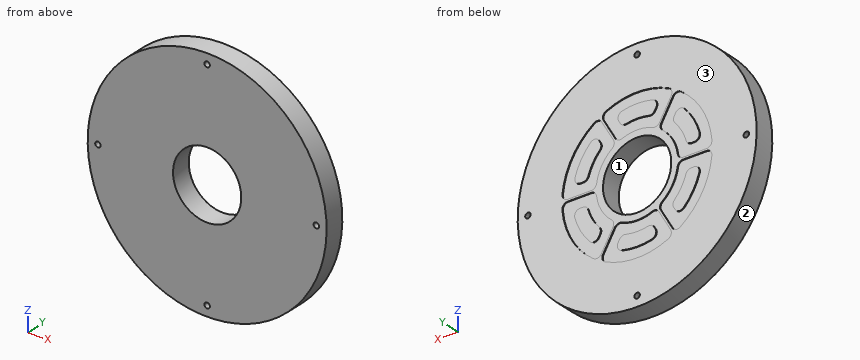
from build123d import *

# Parameters (mm, degrees)
SKETCH2_R           = 175
BOSS_EXTRUDE1_DEPTH = 15
SKETCH3_R           = 4
SKETCH3_R_2         = 50
CUT_EXTRUDE1_DEPTH  = 30
CUT_EXTRUDE3_DEPTH  = 1
CIRPATTERN2_COUNT   = 6


with BuildPart() as part:
    # Sketch2 → Boss-Extrude1 (new, symmetric)
    with BuildSketch(Plane(origin=(0, 0, 0), x_dir=(1, 0, 0), z_dir=(0, 1, 0))):
        with Locations(Location((0, 0, 0), (0, 0, 270))):
            Circle(SKETCH2_R)
    extrude(amount=BOSS_EXTRUDE1_DEPTH, both=True)

    # Sketch3 → Cut-Extrude1 (cut)
    with BuildSketch(Plane(origin=(0, 15, 0), x_dir=(1, 0, 0), z_dir=(0, 1, 0))):
        with Locations(Location((0, 160, 0), (0, 0, 270))):
            Circle(SKETCH3_R)
        with Locations(Location((0, -160, 0), (0, 0, 90))):
            Circle(SKETCH3_R)
        with Locations(Location((-160, 0, 0), (0, 0, 270))):
            Circle(SKETCH3_R)
        with Locations(Location((160, 0, 0), (0, 0, 90))):
            Circle(SKETCH3_R)
        with Locations(Location((0, 0, 0), (0, 0, 270))):
            Circle(SKETCH3_R_2)
    extrude(amount=-CUT_EXTRUDE1_DEPTH, mode=Mode.SUBTRACT)

    # Sketch4 → Cut-Extrude3 (cut)
    with BuildSketch(Plane(origin=(0, 15, 0), x_dir=(1, 0, 0), z_dir=(0, 1, 0))):
        with BuildLine():
            ThreePointArc((-36.613340144, 47.533812423), (-51.737318493, 30.385027154), (-59.347664897, 8.823529412))
            ThreePointArc((-59.347664897, 8.823529412), (-62.036309634, 3.941462028), (-67.260686883, 2))
            Line((-67.260686883, 2), (-101.508620324, 2))
            ThreePointArc((-101.508620324, 2), (-107.436288913, 4.627594105), (-109.470080741, 10.784313725))
            ThreePointArc((-109.470080741, 10.784313725), (-94.99085495, 55.468346611), (-63.19102199, 90.038295963))
            ThreePointArc((-63.19102199, 90.038295963), (-56.868026794, 91.301361412), (-51.667108069, 87.490056256))
            Line((-51.667108069, 87.490056256), (-34.5669156, 57.87165408))
            ThreePointArc((-34.5669156, 57.87165408), (-33.647401917, 52.31816148), (-36.613340144, 47.533812423))
        make_face()
        with BuildLine():
            ThreePointArc((-55.668486055, 64.420646227), (-61.622662682, 68.361129347), (-68.352706691, 65.97656772))
            ThreePointArc((-68.352706691, 65.97656772), (-81.986434608, 47.991921614), (-90.993256658, 27.298850575))
            ThreePointArc((-90.993256658, 27.298850575), (-89.749031081, 20.224584028), (-83.330666624, 17))
            Line((-83.330666624, 17), (-79.14543575, 17))
            ThreePointArc((-79.14543575, 17), (-74.41664671, 18.547205705), (-71.516960015, 22.590361446))
            ThreePointArc((-71.516960015, 22.590361446), (-64.714174788, 37.908779742), (-54.679341331, 51.333903335))
            ThreePointArc((-54.679341331, 51.333903335), (-52.564762349, 55.890540621), (-53.583601177, 60.80951969))
            Line((-53.583601177, 60.80951969), (-55.668486055, 64.420646227))
        make_face(mode=Mode.SUBTRACT)
    cut_extrude3 = extrude(amount=-CUT_EXTRUDE3_DEPTH, mode=Mode.SUBTRACT)

    # CirPattern2: Cut-Extrude3 ×6 about axis
    cirpattern2_axis = Axis((0, 0, 0), (0, 1, 0))
    for i in range(1, CIRPATTERN2_COUNT):
        add(cut_extrude3.rotate(cirpattern2_axis, i * 360 / CIRPATTERN2_COUNT), mode=Mode.SUBTRACT)


solid = part.part
Model file for the job. Use its own axes, mm. Face numbers are marked on the shaded views. Give positions to 0.01 mm unless a question says otherwise; leave off trailing zeros. Write each loop counter-clockwise with the first axis right and the second up, starting at its lowest first coordinate (ties: lowest second). Pieces come first, ordered by that corner, then holes. Notation, with made-up numbers: (-10, 34.5) -> (25, 34.5) arc R16 cw to (25, 64.5) -> close; hole circle Ø1 at (-29.75, 50). An arc over 180 degrees is marked (long way). Write item = value, one per line.
(1) Slice it at A-A, the plane x = 0. Give the number of separate pieces and of enclosed holes in the cut face, then the cut area to 3 significant figures.
Determined:
separate_pieces = 4
enclosed_holes = 0
area = 6,960 mm2
(2) Flat gauge pins, fed straight in: P1, Ø9, axis at x = -160, z = 0, coming from the -Y side; P2, Ø5, axis at y = -8.5, z = -53.5, coming from the -X side; P3, Ø2, axis at x = -86.5, y = 3.5, coming from the -Z side; P4, Ø5, axis at y = -8.5, z = 73, coming from the +X side. Where does each tip first touch, or does it go through?
Determined:
P1 = -15
P2 = -167.4
P3 = -152.69
P4 = 160.17
(3) Slice it at D-D, the plane x = 160. Give the cut face in (y, z).
Determined:
outline = (-15, -70.89) -> (15, -70.89) -> (15, -4) -> (-15, -4) -> close; (-15, 4) -> (15, 4) -> (15, 70.89) -> (-15, 70.89) -> close
(4) Mould opens along X. For the marked faces 1, 2 and 3 say: released by +X, released by -X, zero draft, split by the parting line, or undercut.
Determined:
face_1 = undercut
face_2 = split by the parting line
face_3 = zero draft
(5) Slice it at C-C, the plane y = -4. Give the cut face in (x, z), then the cut area to 3 significant figures.
Determined:
outline = circle Ø350 at (0, 0); hole circle Ø8 at (-160, 0); hole circle Ø100 at (0, 0); hole circle Ø8 at (0, -160); hole circle Ø8 at (0, 160); hole circle Ø8 at (160, 0)
area = 88,200 mm2
(6) Slice it at B-B, the plane z = 38. Give the cut face in (x, y).
Determined:
outline = (-170.82, -15) -> (-32.5, -15) -> (-32.5, 15) -> (-46.43, 15) -> (-46.43, 14) -> (-64.66, 14) -> (-64.66, 15) -> (-87.07, 15) -> (-87.07, 14) -> (-103.23, 14) -> (-103.23, 15) -> (-170.82, 15) -> close; (32.5, -15) -> (170.82, -15) -> (170.82, 15) -> (103.23, 15) -> (103.23, 14) -> (87.07, 14) -> (87.07, 15) -> (64.66, 15) -> (64.66, 14) -> (46.43, 14) -> (46.43, 15) -> (32.5, 15) -> close
(7) Probe line 1 along X through (y, z) = (-3, 0); line 2 along Z through (x, y) = (-33.5, 11.5); line 3 along X through (y, z) = (-5.5, 160). List the from-to ranges inside material, lowest first.
Determined:
line_1 = -175 to -164, -156 to -50, 50 to 156, 164 to 175
line_2 = -171.76 to -37.12, 37.12 to 171.76
line_3 = -70.89 to -4, 4 to 70.89
